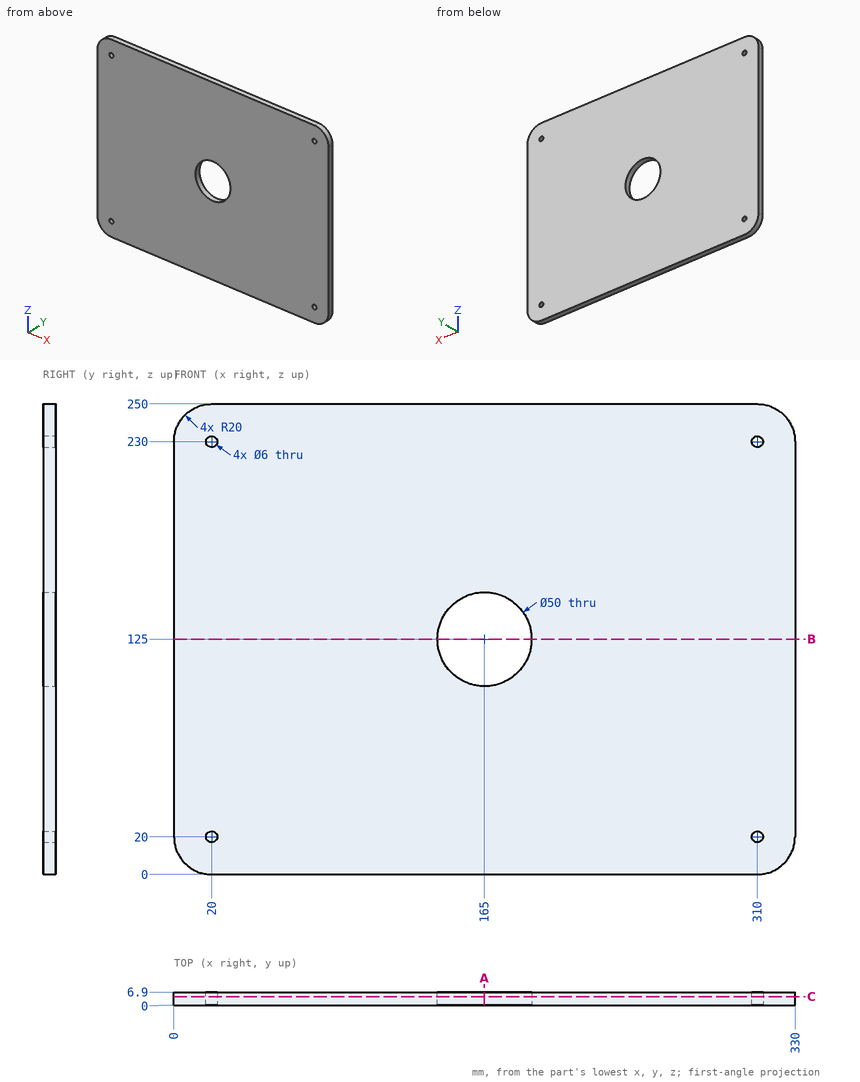
Could you check a few things on this drawing? It's one solid part, dimensions in mm from its lowest x, y, z. Give positions to 0.01 mm unless a question says otherwise; leave off trailing zeros. Order: outer loops, then holes, each group sorted by start corner. A loop starts at its lowest first (then second) coordinate and runs counter-clockwise, first axis right, second up. Notation, with made-up numbers: (16, 75) - (57, 75) arc R25 ccw to (57, 90) - close; hole circle Ø7 at (-26, -6.75). An arc over 180 degrees is marked (long way). One line per item, written item: value. Start each with the question number.
1. If I drill on probe 1 along Z at (x, y) = (20, 4.75); probe 2 along X at (y, z) = (1.75, 230); probe 3 along X at (y, z) = (2.25, 125), over which ranges is the centre line in solid material (lowest first)?
2. Imagine slicing it at A-A on x = 165. List the corners of the cut face in (y, z) for me.
3. Imagine slicing it at B-B on z = 125. List the corners of the cut face in (x, y) for me, plus the area to 3 significant figures.
4. Imagine slicing it at C-C on y = 4.75. List the corners of the cut face in (x, z) for me, plus the area to 3 significant figures.
Values:
1. probe 1: 0 to 17, 23 to 227, 233 to 250
1. probe 2: 0 to 17, 23 to 307, 313 to 330
1. probe 3: 0 to 140, 190 to 330
2. outline: (0, 0) - (6.9, 0) - (6.9, 100) - (0, 100) - close; (0, 150) - (6.9, 150) - (6.9, 250) - (0, 250) - close
3. outline: (0, 0) - (140, 0) - (140, 6.9) - (0, 6.9) - close; (190, 0) - (330, 0) - (330, 6.9) - (190, 6.9) - close
3. area: 1,930 mm²
4. outline: (0, 20) arc R20 ccw to (20, 0) - (310, 0) arc R20 ccw to (330, 20) - (330, 230) arc R20 ccw to (310, 250) - (20, 250) arc R20 ccw to (0, 230) - close; hole circle Ø6 at (20, 20); hole circle Ø6 at (20, 230); hole circle Ø50 at (165, 125); hole circle Ø6 at (310, 20); hole circle Ø6 at (310, 230)
4. area: 80,100 mm²
